Check sheet for the modelled part. Datum: model origin and axes. Units: mm. A direction names the side the tool comes from. Coordinates: 2 decimals unless noted, no trailing zeros. Loops run counter-clockwise (first coordinate to the right, second up) from the corner with the lowest first, then second, coordinate; pieces in that order, holes last. Notation, with made-up numbers: (-24.5, -37.5) - (-14.5, -37.5) arc R20 ccw to (-14.5, -19.5) - close; hole circle Ø9 at (-24.75, -11). An arc over 180 degrees is marked (long way). Write each question's results on one line, items separated by ' | '. Start each with the question number.
1. Gauge pin test, flat ends, axial feed: P1, Ø1, axis at y = 7.5, z = -1, coming from the -X side; P2, Ø2, axis at x = -32, z = -2.5, coming from the +Y side (3 decimals); P3, Ø1.7, axis at y = 16, z = 1, coming from the -X side; P4, Ø2, axis at x = -3, y = -18, coming from the -Z side. Record the tip position at first contact, or that the pin passes through.
2. Cross-section at A-A (y = 27). Record the cut outline in (x, z).
3. Tool access check on faces 1 (the face through (-32, 3.175, -2)), 2 (the face through (-30.861, 0, -3)), 3 (the face through (-32, -3.175, -2)), 4 (the face through (-32, 0, -5.588)). Record the directions out of +Z, -Z, +X, -X, +Y, -Y that give a thin tool (end or side, any length) a straight path to the whole face; none if there is none.
4. Thickness scan on line 1 (Z direction, x = 6.5, y = -37.5); line 2 (X direction, y = -29.5, z = 1); line 3 (X direction, y = 2, z = -2). Record the ranges inside material, lowest first. Write a range as [from, to].
5. Cross-section at B-B (z = -2.75). Record the cut outline in (x, y) (3 decimals).
```python
from build123d import *

# Parameters (mm, degrees)
F0_W     = 61.722
F0_H     = 86.36
F1_DEPTH = 1.524
F2_W     = 6.35
F2_H     = 3.048
F3_DEPTH = 1.9304
F4_W     = 1.9304
F4_H     = 6.35
F5_DEPTH = 4.064


with BuildPart() as f1:
    # F0 (on Top) → F1 (new body)
    with BuildSketch(Plane.XY):
        Rectangle(F0_W, F0_H)
    extrude(amount=F1_DEPTH)

    # F2 (on face) → F3 (join)
    with BuildSketch(Plane(origin=(-30.861, 0, 0), x_dir=(0, -1, 0), z_dir=(-1, 0, 0))):
        Rectangle(F2_W, F2_H)
    extrude(amount=F3_DEPTH)

    # F4 (on face) → F5 (join)
    with BuildSketch(Plane(origin=(0, 0, -1.524), x_dir=(1, 0, 0), z_dir=(0, 0, -1))):
        with Locations((-31.8262, 0)):
            Rectangle(F4_W, F4_H)
    extrude(amount=F5_DEPTH)


solid = f1.part
```
Established:
1) P1: through | P2: y = 3.175 | P3: x = -30.86 | P4: z = 0
2) outline: (-30.86, 0) - (30.86, 0) - (30.86, 1.52) - (-30.86, 1.52) - close
3) face 1: +Z, -Z, -X, +Y | face 2: -Z, +X, +Y, -Y | face 3: +Z, -Z, -X, -Y | face 4: -Z, +X, -X, +Y, -Y
4) line 1: [0, 1.52] | line 2: [-30.86, 30.86] | line 3: [-32.79, -30.86]
5) outline: (-32.791, -3.175) - (-30.861, -3.175) - (-30.861, 3.175) - (-32.791, 3.175) - close
